Read the model definition and answer for the solid it produces. Units are mm, in the model's axes. Face numbers are marked on the shaded views. A direction names the side the tool comes from. Give positions to 0.01 mm unless a question says otherwise; leave off trailing zeros. Order: outer loops, then holes, each group sorted by start corner. A loop starts at its lowest first (then second) coordinate and runs counter-clockwise, first axis right, second up. Notation, with made-up numbers: (35.25, -29.75) -> (42.25, -29.75) arc R23 ccw to (42.25, 2.25) -> close; hole circle Ø3 at (18.25, 41.25). An arc over 180 degrees is marked (long way). Use one line per item in the form item = value.
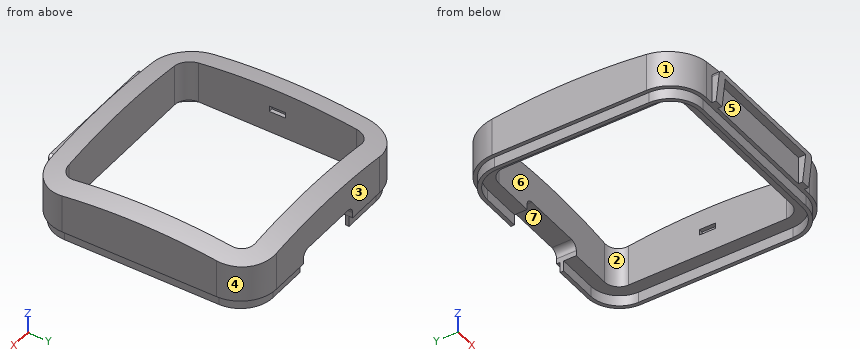
```python
from build123d import *

# Parameters (mm, degrees)
PAD_DEPTH       = 15
SKETCH_W        = 4.5
SKETCH_H        = 1.6
POCKET_DEPTH    = 1.1
POCKET001_DEPTH = 5.499984
PAD001_DEPTH    = 5
POCKET002_DEPTH = 50.750998
PAD002_DEPTH    = 3


with BuildPart() as limit_walls:
    # Sketch002 → Revolution001 (revolve)
    with BuildSketch(Plane.YZ):
        with BuildLine():
            ThreePointArc((60, -10.940263), (30.494628, -2.757429), (0, 0))
            Line((0, 10), (0, 0))
            ThreePointArc((63.529412, -1.583808), (32.28843, 7.08037), (0, 10))
            Line((63.529412, -1.583808), (60, -10.940263))
        make_face()
    revolve(axis=Axis((0, 0, 0), (0, 0, 1)))


with BuildPart() as cut:
    # Sketch001 → Pad (new body)
    with BuildSketch(Plane.XY.offset(-15)):
        with BuildLine():
            Line((-21.499971, 31.499984), (21.499999, 31.499984))
            ThreePointArc((31.499998, 21.499986), (28.571066, 28.571052), (21.499999, 31.499984))
            Line((31.499998, 21.499986), (31.499998, -21.499984))
            ThreePointArc((21.499971, -31.499984), (28.571056, -28.571062), (31.499998, -21.499984))
            Line((-21.499999, -31.499984), (21.499971, -31.499984))
            ThreePointArc((-31.500002, -21.499984), (-28.571069, -28.571053), (-21.499999, -31.499984))
            Line((-31.500002, 21.499986), (-31.500002, -21.499984))
            ThreePointArc((-21.499971, 31.499984), (-28.571058, 28.571064), (-31.500002, 21.499986))
        make_face()
        with BuildLine():
            Line((-22, 26), (22, 26))
            ThreePointArc((26, 22), (24.828427, 24.828427), (22, 26))
            Line((26, 22), (26, -22))
            ThreePointArc((22, -26), (24.828427, -24.828427), (26, -22))
            Line((-22, -26), (22, -26))
            ThreePointArc((-26, -21.99998), (-24.828434, -24.82842), (-22, -26))
            Line((-26, 22.000021), (-26, -21.99998))
            ThreePointArc((-22, 26), (-24.82842, 24.828435), (-26, 22.000021))
        make_face(mode=Mode.SUBTRACT)
    extrude(amount=PAD_DEPTH)

    # Sketch (on Face9 of Pad) → Pocket (cut)
    with BuildSketch(Plane.YZ.offset(-26)):
        with Locations((0, -8.2)):
            Rectangle(SKETCH_W, SKETCH_H)
    pocket = extrude(amount=-POCKET_DEPTH, mode=Mode.SUBTRACT)

    # Mirrored: Pocket across YZ
    add(pocket.mirror(Plane.YZ), mode=Mode.SUBTRACT)

    # Sketch003 (on Face2 of Mirrored) → Pocket001 (cut)
    with BuildSketch(Plane(origin=(0, 31.499984, 0), x_dir=(-1, 0, 0), z_dir=(0, 1, 0))):
        with BuildLine():
            Line((-10.25, -15), (-10.25, -13.500001))
            ThreePointArc((-8.249997, -11.5), (-9.664212, -12.085786), (-10.25, -13.500001))
            Line((-8.249997, -11.5), (8.249997, -11.5))
            ThreePointArc((10.249996, -13.500001), (9.66421, -12.085787), (8.249997, -11.5))
            Line((10.25, -15), (10.249996, -13.500001))
            Line((-10.25, -15), (10.25, -15))
        make_face()
    extrude(amount=-POCKET001_DEPTH, mode=Mode.SUBTRACT)

    # Sketch004 (on Face13 of Pocket001) → Pad001 (join)
    with BuildSketch(Plane.XZ.offset(31.499984)):
        with BuildLine():
            Line((-19.25, -15), (-19.25, -7.25))
            ThreePointArc((-18, -6), (-18.883883, -6.366117), (-19.25, -7.25))
            Line((-18, -6), (18, -6))
            ThreePointArc((19.25, -7.25), (18.883883, -6.366117), (18, -6))
            Line((19.25, -15), (19.25, -7.25))
            Line((16.75, -15), (19.25, -15))
            Line((16.75, -15), (16.75, -7.25))
            Line((-16.75, -7.25), (16.75, -7.25))
            Line((-16.75, -15), (-16.75, -7.25))
            Line((-19.25, -15), (-16.75, -15))
        make_face()
    extrude(amount=PAD001_DEPTH)

    # Sketch005 (on Face27 of Pad001) → Pocket002 (cut, through all)
    with BuildSketch(Plane(origin=(-19.25, 0, 0), x_dir=(0, -1, 0), z_dir=(-1, 0, 0))):
        Polygon((33.699984, -6), (32.699984, -15), (36.499984, -15), (36.499984, -6), align=None)
    extrude(amount=-POCKET002_DEPTH, mode=Mode.SUBTRACT)

    # Sketch006 (on Face4 of Pocket002) → Pad002 (join)
    with BuildSketch(Plane(origin=(0, 0, -15), x_dir=(1, 0, 0), z_dir=(0, 0, -1))):
        with BuildLine():
            Line((-21.499999, 30.499984), (21.499999, 30.499984))
            ThreePointArc((30.499997, 21.499984), (27.863964, 27.86395), (21.499999, 30.499984))
            Line((30.499997, 21.499984), (30.499997, -21.499984))
            ThreePointArc((21.500015, -30.499984), (27.86397, -27.863944), (30.499997, -21.499984))
            Line((21.500015, -30.499984), (10.25, -30.499984))
            Line((10.25, -29.499984), (10.25, -30.499984))
            Line((21.500015, -29.499984), (10.25, -29.499984))
            ThreePointArc((21.500015, -29.499984), (27.156863, -27.156837), (29.499997, -21.499984))
            Line((29.499997, 21.499984), (29.499997, -21.499984))
            ThreePointArc((29.499997, 21.499984), (27.156857, 27.156843), (21.499999, 29.499984))
            Line((-21.499999, 29.499984), (21.499999, 29.499984))
            ThreePointArc((-21.499999, 29.499984), (-27.156852, 27.156838), (-29.499997, 21.499984))
            Line((-29.499997, 21.499984), (-29.499997, -21.499984))
            ThreePointArc((-29.499997, -21.499984), (-27.156863, -27.156837), (-21.500016, -29.499984))
            Line((-21.500016, -29.499984), (-10.25, -29.499984))
            Line((-10.25, -30.499984), (-10.25, -29.499984))
            Line((-21.500015, -30.499984), (-10.25, -30.499984))
            ThreePointArc((-30.499997, -21.499984), (-27.86397, -27.863944), (-21.500015, -30.499984))
            Line((-30.499997, 21.499984), (-30.499997, -21.499984))
            ThreePointArc((-21.499999, 30.499984), (-27.863964, 27.86395), (-30.499997, 21.499984))
        make_face()
    extrude(amount=PAD002_DEPTH)

    # Cut: cut limit_walls
    add(limit_walls.part, mode=Mode.SUBTRACT)


solid = cut.part
```
Item 1: Straight lines are drawn through the part: L1, parallel to Y at x = 20.5, z = -16.25; L2, parallel to Y at x = 5.5, z = -3.5. For each, find the intervals that lie inside material, in ascending order. Write a range as from..to.
Checks:
L1 = -30.5..-29.5, 29.5..30.5
L2 = -31.5..-26, 26..31.5
Item 2: The part is cut by section B-B on z = -12.25. Give the vertices of the cut face in (x, y).
Checks:
outline = (-31.5, -21.5) arc R10 ccw to (-21.5, -31.5) -> (-19.25, -31.5) -> (-19.25, -33.01) -> (-16.75, -33.01) -> (-16.75, -31.5) -> (16.75, -31.5) -> (16.75, -33.01) -> (19.25, -33.01) -> (19.25, -31.5) -> (21.5, -31.5) arc R10 ccw to (31.5, -21.5) -> (31.5, 21.5) arc R10 ccw to (21.5, 31.5) -> (9.81, 31.5) -> (9.81, 26) -> (22, 26) arc R4 cw to (26, 22) -> (26, -22) arc R4 cw to (22, -26) -> (-22, -26) arc R4 cw to (-26, -22) -> (-26, 22) arc R4 cw to (-22, 26) -> (-9.81, 26) -> (-9.81, 31.5) -> (-21.5, 31.5) arc R10 ccw to (-31.5, 21.5) -> close
Item 3: The part is cut by section A-A on z = -16.5. Give the vertices of the cut face in (x, y).
Checks:
outline = (-30.5, -21.5) arc R9 ccw to (-21.5, -30.5) -> (21.5, -30.5) arc R9 ccw to (30.5, -21.5) -> (30.5, 21.5) arc R9 ccw to (21.5, 30.5) -> (10.25, 30.5) -> (10.25, 29.5) -> (21.5, 29.5) arc R8 cw to (29.5, 21.5) -> (29.5, -21.5) arc R8 cw to (21.5, -29.5) -> (-21.5, -29.5) arc R8 cw to (-29.5, -21.5) -> (-29.5, 21.5) arc R8 cw to (-21.5, 29.5) -> (-10.25, 29.5) -> (-10.25, 30.5) -> (-21.5, 30.5) arc R9 ccw to (-30.5, 21.5) -> close
Item 4: Which of the six approach directions +Z, -Z, +X, -X, +Y, -Y give full straight-line access (tool end or side, diameter ignored) to the marked faces 5, 6 and 7?
Checks:
face_5 = -Z, -Y
face_6 = +Z, -Z
face_7 = -Z, +Y
Item 5: Determine the mould class of the marked faces 1, 2, 3 and 4 for opening direction X: +X half, -X half, draft (parallel to the pull), parting line (faces both ways), or undercut.
Checks:
face_1 = -X half
face_2 = undercut
face_3 = draft
face_4 = +X half
Item 6: Given pin 1 Ø1.5 at (x, z) = (-16.5, -16.5) entering from -Y; pin 2 Ø6 at (x, z) = (-10.5, -15) entering from -Y; pin 3 Ø2 at (y, z) = (27.5, -16.5) entering from -X, each flat-ended and moving along its own axis, determine where each tip first touches the part or whether it passes through.
Checks:
pin_1 = -30.5
pin_2 = -31.5
pin_3 = -28.98
